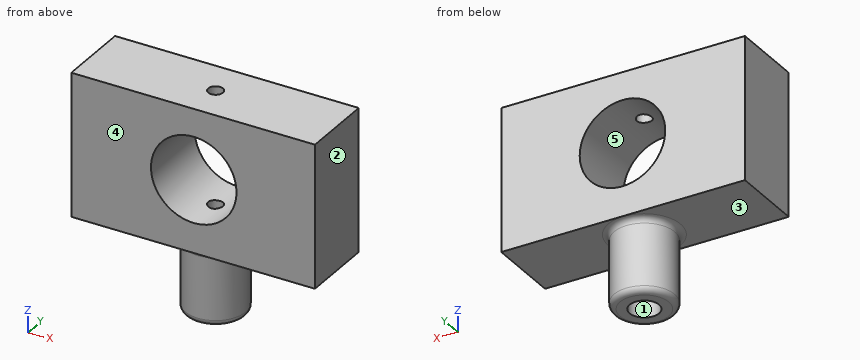
```python
from build123d import *

# Parameters (mm, degrees)
F0_W           = 82.594938
F0_H           = 48.417722
F1_DEPTH       = 12.5
F2_R           = 14.500066
F3_DEPTH       = 25.001
F4_R           = 10.249702
F5_DEPTH       = 25
F6_R           = 2
F8_D           = 5
F8_CBORE_D     = 10
F8_CBORE_DEPTH = 10


with BuildPart() as f1:
    # F0 (on Front) → F1 (new body, symmetric)
    with BuildSketch(Plane.XZ):
        with Locations((-0.213608, -0.356012)):
            Rectangle(F0_W, F0_H)
    extrude(amount=F1_DEPTH, both=True)

    # F2 (on face) → F3 (cut, through all)
    with BuildSketch(Plane.XZ.offset(12.5)):
        Circle(F2_R)
    extrude(amount=-F3_DEPTH, mode=Mode.SUBTRACT)

    # F4 (on face) → F5 (join)
    with BuildSketch(Plane(origin=(0, 0, -24.564873), x_dir=(1, 0, 0), z_dir=(0, 0, -1))):
        Circle(F4_R)
    extrude(amount=F5_DEPTH)

    # F6
    f6_edges = [f1.edges().sort_by_distance(p)[0] for p in [
        (-10.249702, 0, -49.564873),
        (10.249702, 0, -37.064873),
        (-10.249702, 0, -24.564873),
    ]]
    fillet(f6_edges, radius=F6_R)

    # F8 (through all)
    with Locations(Plane(origin=(0, 0, -49.564873), x_dir=(1, 0, 0), z_dir=(0, 0, -1))):
        with Locations((0, 0)):
            CounterBoreHole(F8_D / 2, F8_CBORE_D / 2, F8_CBORE_DEPTH)


solid = f1.part
```
CAD build for the part. Positions are in the model's coordinates, mm. Face numbers are marked on the shaded views. A direction names the side the tool comes from. Round coordinates to 2 decimals unless told otherwise and drop trailing zeros. Loops run counter-clockwise (first coordinate to the right, second up) from the corner with the lowest first, then second, coordinate; pieces in that order, holes last. Notation, with made-up numbers: (37.5, 29) - (79.5, 29) arc R16 ccw to (79.5, 60) - close; hole circle Ø3 at (-12.75, 74). An arc over 180 degrees is marked (long way). Return JSON: item names as keys, results as strings. Group by question number.
Q1. Band-saw the part on C-C on y = 0. Give the cut face in (x, z), plus the area to 3 significant figures.
Q2. Drill centre lines: line 1 along Y through (x, z) = (0, 18.75); line 2 along X through (y, z) = (10.5, 0.5); line 3 along Y through (x, z) = (0, -44). Where is each one in solid material? Low to high. Write a range as [from, to].
Q3. Two-plate mould, pull along Z, no slides. Class the marked faces 3, 4 and 5: +Z half, -Z half, draft (parallel to the pull), parting line (faces both ways), or undercut.
Q4. Band-saw the part on D-D on z = -33. Give the cut face in (x, y).
Q5. Band-saw the part on A-A on z = 0. Give the cut face in (x, y), plus the area to 3 significant figures.
Q6. Tool access for the marked faces 1 and 2: list every direction of +Z, -Z, +X, -X, +Y, -Y with a clear straight run to the whole face (end or side of a thin tool).
Q7. Band-saw the part on B-B on x = 0. Give the cut face in (y, z), plus the area to 3 significant figures.
Q8. Flat gauge pins, fed straight in: pin 1 Ø3 at (x, y) = (20.5, -2.5) entering from -Z; pin 2 Ø2 at (y, z) = (-2, -34) entering from +X; pin 3 Ø12.5 at (x, y) = (14.5, -4) entering from -Z. Where does each tip first touch, or does it go through?
Solutions:
{
 "1": {"outline": "(-41.51, -24.56) - (-12.25, -24.56) arc R2 cw to (-10.25, -26.56) - (-10.25, -47.56) arc R2 ccw to (-8.25, -49.56) - (-5, -49.56) - (-5, -39.56) - (-2.5, -39.56) - (-2.5, -14.28) arc R14.5 cw to (-2.5, 14.28) - (-2.5, 23.85) - (-41.51, 23.85) - close; (2.5, -39.56) - (5, -39.56) - (5, -49.56) - (8.25, -49.56) arc R2 ccw to (10.25, -47.56) - (10.25, -26.56) arc R2 cw to (12.25, -24.56) - (41.08, -24.56) - (41.08, 23.85) - (2.5, 23.85) - (2.5, 14.28) arc R14.5 cw to (2.5, -14.28) - close", "area": "3,580 mm^2"},
 "2": {"line 1": "y = [-12.5, -2.5], [2.5, 12.5]", "line 2": "x = [-41.51, -14.49], [14.49, 41.08]", "line 3": "y = [-10.25, -5], [5, 10.25]"},
 "3": {"face 3": "-Z half", "face 4": "draft", "face 5": "undercut"},
 "4": {"outline": "circle Ø20.5 at (0, 0); hole circle Ø5 at (0, 0)"},
 "5": {"outline": "(-41.51, -12.5) - (-14.5, -12.5) - (-14.5, 12.5) - (-41.51, 12.5) - close; (14.5, -12.5) - (41.08, -12.5) - (41.08, 12.5) - (14.5, 12.5) - close", "area": "1,340 mm^2"},
 "6": {"face 1": "-Z", "face 2": "+Z, -Z, +X, +Y, -Y"},
 "7": {"outline": "(-12.5, -24.56) - (-12.25, -24.56) arc R2 cw to (-10.25, -26.56) - (-10.25, -47.56) arc R2 ccw to (-8.25, -49.56) - (-5, -49.56) - (-5, -39.56) - (-2.5, -39.56) - (-2.5, -14.5) - (-12.5, -14.5) - close; (-12.5, 14.5) - (-2.5, 14.5) - (-2.5, 23.85) - (-12.5, 23.85) - close; (2.5, -39.56) - (5, -39.56) - (5, -49.56) - (8.25, -49.56) arc R2 ccw to (10.25, -47.56) - (10.25, -26.56) arc R2 cw to (12.25, -24.56) - (12.5, -24.56) - (12.5, -14.5) - (2.5, -14.5) - close; (2.5, 14.5) - (12.5, 14.5) - (12.5, 23.85) - (2.5, 23.85) - close", "area": "726 mm^2"},
 "8": {"pin 1": "stops at z = -24.56", "pin 2": "stops at x = 10.2", "pin 3": "stops at z = -49.49"}
}
